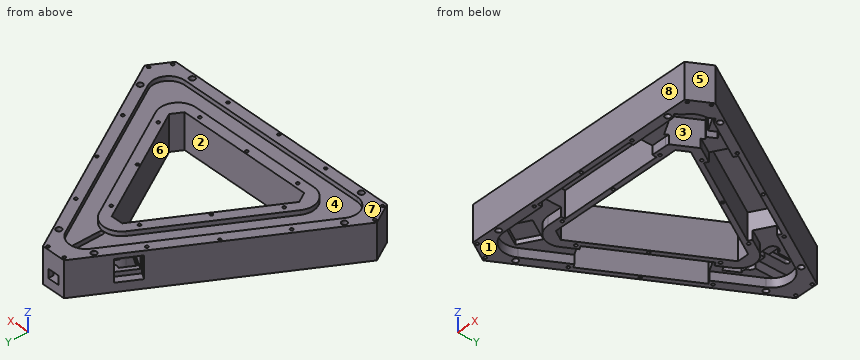
from build123d import *

# Parameters (mm, degrees)
PAD_DEPTH             = 24
POCKET_DEPTH          = 3
SKETCH002_W           = 70
SKETCH002_H           = 18.5
POCKET001_DEPTH       = 18
POLARPATTERN_COUNT    = 3
POCKET002_DEPTH       = 6
CHAMFER_SIZE          = 8
FILLET_R              = 13
FILLET001_R           = 11
CHAMFER001_SIZE       = 16.1
FILLET002_R           = 11
FILLET003_R           = 12
POCKET003_DEPTH       = 6
POCKET004_DEPTH       = 18
POCKET005_DEPTH       = 21.001
SKETCH007_W           = 15.5
SKETCH007_H           = 15
POCKET006_DEPTH       = 5
SKETCH010_W           = 13.6
SKETCH010_H           = 9
POCKET009_DEPTH       = 15.5
POCKET010_DEPTH       = 3
SKETCH012_R           = 1.85
SKETCH012_R_2         = 0.99
POCKET011_DEPTH       = 498.0492855781
POLARPATTERN001_COUNT = 3
POCKET012_DEPTH       = 12
POCKET013_DEPTH       = 3
POCKET014_DEPTH       = 3
FILLET004_R           = 0.6
FILLET005_R           = 2.6


with BuildPart() as part:
    # Sketch → Pad (new body)
    with BuildSketch(Plane.XY):
        Polygon((0, 112.2094915052), (-97.1762701892, -56.1047457526), (97.1762701892, -56.1047457526), align=None)
        Polygon((0, 62.2094915052), (-53.875, -31.1047457526), (53.875, -31.1047457526), align=None, mode=Mode.SUBTRACT)
    extrude(amount=PAD_DEPTH)

    # Sketch001 (on Face8 of Pad) → Pocket (cut)
    with BuildSketch(Plane.XY.offset(24)):
        Polygon((0, 98.2094915052), (-85.0519145362, -49.1047457526), (85.0519145362, -49.1047457526), align=None)
        Polygon((0, 76.2094915052), (-65.999355653, -38.1047457526), (65.999355653, -38.1047457526), align=None, mode=Mode.SUBTRACT)
    extrude(amount=-POCKET_DEPTH, mode=Mode.SUBTRACT)

    # Sketch002 (on Face4 of Pocket) → Pocket001 (cut)
    with BuildSketch(Plane(origin=(0, 0, 0), x_dir=(1, 0, 0), z_dir=(0, 0, -1))):
        with Locations((0, 43.6047457526)):
            Rectangle(SKETCH002_W, SKETCH002_H)
    pocket001 = extrude(amount=-POCKET001_DEPTH, mode=Mode.SUBTRACT)

    # PolarPattern: Pocket001 ×3 about axis
    polarpattern_axis = Axis((0, 0, 0), (0, 0, -1))
    for i in range(1, POLARPATTERN_COUNT):
        add(pocket001.rotate(polarpattern_axis, i * 360 / POLARPATTERN_COUNT), mode=Mode.SUBTRACT)

    # Sketch003 (on Face4 of PolarPattern) → Pocket002 (cut)
    with BuildSketch(Plane(origin=(0, 0, 0), x_dir=(1, 0, 0), z_dir=(0, 0, -1))):
        Polygon((0, -100.2094915052), (86.7839653438, 50.1047457526), (-86.7839653438, 50.1047457526), align=None)
        Polygon((0, -74.2094915052), (64.2673048454, 37.1047457526), (-64.2673048454, 37.1047457526), align=None, mode=Mode.SUBTRACT)
    extrude(amount=-POCKET002_DEPTH, mode=Mode.SUBTRACT)

    # Chamfer
    chamfer_edges = [part.edges().sort_by_distance(p)[0] for p in [
        (-53.875, -31.104746, 12),
        (53.875, -31.104746, 12),
        (0, 62.209492, 12),
    ]]
    chamfer(chamfer_edges, length=CHAMFER_SIZE)

    # Fillet
    fillet_edges = [part.edges().sort_by_distance(p)[0] for p in [
        (0, 100.209492, 3),
        (-86.783965, -50.104746, 3),
        (86.783965, -50.104746, 3),
    ]]
    fillet(fillet_edges, radius=FILLET_R)

    # Fillet001
    fillet001_edges = [part.edges().sort_by_distance(p)[0] for p in [
        (0, 74.209492, 3),
        (64.267305, -37.104746, 3),
        (-64.267305, -37.104746, 3),
    ]]
    fillet(fillet001_edges, radius=FILLET001_R)

    # Chamfer001
    chamfer001_edges = [part.edges().sort_by_distance(p)[0] for p in [
        (97.17627, -56.104746, 12),
        (0, 112.209492, 12),
        (-97.17627, -56.104746, 12),
    ]]
    chamfer(chamfer001_edges, length=CHAMFER001_SIZE)

    # Fillet002
    fillet002_edges = [part.edges().sort_by_distance(p)[0] for p in [
        (0, 98.209492, 22.5),
        (-85.051915, -49.104746, 22.5),
        (85.051915, -49.104746, 22.5),
    ]]
    fillet(fillet002_edges, radius=FILLET002_R)

    # Fillet003
    fillet003_edges = [part.edges().sort_by_distance(p)[0] for p in [
        (65.999356, -38.104746, 22.5),
        (0, 76.209492, 22.5),
        (-65.999356, -38.104746, 22.5),
    ]]
    fillet(fillet003_edges, radius=FILLET003_R)

    # Sketch004 (on Face60 of Fillet003) → Pocket003 (cut)
    with BuildSketch(Plane(origin=(0, 0, 6), x_dir=(1, 0, 0), z_dir=(0, 0, -1))):
        Polygon((-8.75, -71.2664825043), (8.75, -71.2664825043), (8.75, -94.7664825043), (4, -94.7664825043), (4, -98.2664825043), (-4, -98.2664825043), (-4, -94.7664825043), (-8.75, -94.7664825043), align=None)
    extrude(amount=-POCKET003_DEPTH, mode=Mode.SUBTRACT)

    # Sketch005 (on Face29 of Pocket003) → Pocket004 (cut)
    with BuildSketch(Plane(origin=(0, 0, 0), x_dir=(1, 0, 0), z_dir=(0, 0, -1))):
        Polygon((46.1715988394, 38.9547457526), (68.6882593378, 51.9547457526), (79.3382593378, 33.508404652), (56.8215988394, 20.508404652), align=None)
    extrude(amount=-POCKET004_DEPTH, mode=Mode.SUBTRACT)

    # Sketch006 (on Face1 of Pocket004) → Pocket005 (cut, through all)
    with BuildSketch(Plane.XY.offset(21)):
        with BuildLine():
            ThreePointArc((1.5, 85.0404521425), (0, 86.5404521425), (-1.5, 85.0404521425))
            Line((-1.5, 85.0404521425), (-1.5, 66.0404521425))
            ThreePointArc((-1.5, 66.0404521425), (0, 64.5404521425), (1.5, 66.0404521425))
            Line((1.5, 85.0404521425), (1.5, 66.0404521425))
        make_face()
    extrude(amount=-POCKET005_DEPTH, mode=Mode.SUBTRACT)

    # Sketch007 (on Face24 of Pocket005) → Pocket006 (cut)
    with BuildSketch(Plane(origin=(-48.5881350946, 28.0523728763, 0), x_dir=(-0.5, -0.8660254038, 0), z_dir=(-0.8660254038, 0.5, 0))):
        with Locations((-47.3262701892, 13.5)):
            Rectangle(SKETCH007_W, SKETCH007_H)
    extrude(amount=-POCKET006_DEPTH, mode=Mode.SUBTRACT)

    # Sketch010 (on Face79 of Pocket006) → Pocket009 (cut)
    with BuildSketch(Plane(origin=(-44.2580080757, 25.5523728763, 0), x_dir=(-0.5, -0.8660254038, 0), z_dir=(-0.8660254038, 0.5, 0))):
        with Locations((-47.3262701892, 13.5)):
            Rectangle(SKETCH010_W, SKETCH010_H)
    extrude(amount=-POCKET009_DEPTH, mode=Mode.SUBTRACT)

    # Sketch011 (on Face21 of Pocket009) → Pocket010 (cut)
    with BuildSketch(Plane(origin=(0, 0, 6), x_dir=(1, 0, 0), z_dir=(0, 0, -1))):
        Polygon((-21.0413798427, -59.7570681827), (-11.6817654684, -54.3532923042), (-6.658482036, -63.0538744299), (-16.0180964103, -68.4576503084), align=None)
    extrude(amount=-POCKET010_DEPTH, mode=Mode.SUBTRACT)

    # Sketch012 (on Face54 of Pocket010) → Pocket011 (cut, through all)
    with BuildSketch(Plane(origin=(0, 0, 0), x_dir=(1, 0, 0), z_dir=(0, 0, -1))):
        with Locations((-13.5, -82.7032108255)):
            Circle(SKETCH012_R)
        with Locations((13.5, -82.7032108255)):
            Circle(SKETCH012_R)
        with Locations((-6.25, -96.5164825043)):
            Circle(SKETCH012_R_2)
        with Locations((6.25, -96.5164825043)):
            Circle(SKETCH012_R_2)
        with Locations((-27.2463245869, -59.0174730012)):
            Circle(SKETCH012_R_2)
        with Locations((-47.1862074814, -27.2405827309)):
            Circle(SKETCH012_R_2)
        with Locations((-64.7337931796, 5.9127272486)):
            Circle(SKETCH012_R_2)
        with Locations((-10.791841915, -49.5174730012)):
            Circle(SKETCH012_R_2)
        with Locations((-28.3394276132, -16.3641630217)):
            Circle(SKETCH012_R_2)
        with Locations((-48.2793105078, 15.4127272487)):
            Circle(SKETCH012_R_2)
    pocket011 = extrude(amount=-POCKET011_DEPTH, mode=Mode.SUBTRACT)

    # PolarPattern001: Pocket011 ×3 about axis
    polarpattern001_axis = Axis((0, 0, 0), (0, 0, -1))
    for i in range(1, POLARPATTERN001_COUNT):
        add(pocket011.rotate(polarpattern001_axis, i * 360 / POLARPATTERN001_COUNT), mode=Mode.SUBTRACT)

    # Sketch013 (on Face132 of PolarPattern001) → Pocket012 (cut)
    with BuildSketch(Plane(origin=(0, 0, 6), x_dir=(1, 0, 0), z_dir=(0, 0, -1))):
        Polygon((58.553649647, 21.508404652), (63.3167893678, 24.258404652), (66.3167893678, 19.0622522293), (61.553649647, 16.3122522293), align=None)
    extrude(amount=-POCKET012_DEPTH, mode=Mode.SUBTRACT)

    # Sketch014 (on Face127 of Pocket012) → Pocket013 (cut)
    with BuildSketch(Plane(origin=(0, 0, 6), x_dir=(1, 0, 0), z_dir=(0, 0, -1))):
        Polygon((-74.3478338252, 33.3748379063), (-65.8478338252, 48.0972697706), (-52.8574527684, 40.5972697706), (-61.3574527684, 25.8748379063), align=None)
    extrude(amount=-POCKET013_DEPTH, mode=Mode.SUBTRACT)

    # Sketch015 (on Face21 of Pocket013) → Pocket014 (cut)
    with BuildSketch(Plane(origin=(0, 0, 6), x_dir=(1, 0, 0), z_dir=(0, 0, -1))):
        with BuildLine():
            ThreePointArc((-8.75, -64.2614128894), (-12.2525348074, -67.7639476968), (-8.75, -71.2664825043))
            Line((-8.75, -71.2664825043), (8.73, -71.2664825043))
            ThreePointArc((8.73, -71.2664825043), (12.2325348074, -67.7639476968), (8.73, -64.2614128894))
            Line((-8.75, -64.2614128894), (8.73, -64.2614128894))
        make_face()
    extrude(amount=-POCKET014_DEPTH, mode=Mode.SUBTRACT)

    # Fillet004
    fillet004_edges = [part.edges().sort_by_distance(p)[0] for p in [
        (-8.75, 64.261413, 7.5),
    ]]
    fillet(fillet004_edges, radius=FILLET004_R)

    # Fillet005
    fillet005_edges = [part.edges().sort_by_distance(p)[0] for p in [
        (-11.783284, 66.01268, 7.5),
    ]]
    fillet(fillet005_edges, radius=FILLET005_R)


solid = part.part
Input: part model. Units: mm. Frame: model coordinates. Face numbers are marked on the shaded views. A direction names the side the tool comes from. Coordinates: 2 decimals unless noted, no trailing zeros. Write each loop counter-clockwise with the first axis right and the second up, starting at its lowest first coordinate (ties: lowest second). Pieces come first, ordered by that corner, then holes. Notation, with made-up numbers: M 10.5,-19.5 L 36.5,-19.5 A29 ccw 36.5,11.5 Z; hole C 22,-2.75 d11. An arc over 180 degrees is marked long. Answer as a JSON object with one key per item and string values. Group by question number.
(1) Set-up query: the marked faces 1, 2, 3, 4 and 5. Return all of +Z, -Z, +X, -X, +Y, -Y with unobstructed straight access to the full face (end or side cutting, diameter ignored); none if empty.
(2) Section A-A on x = -41.5. Output: boundary loops of the cut face in (y, z).
(3) Contact query for flat-ended pins moving along their axis: P1, Ø8, axis at y = 36.5, z = 6, coming from the +X side; P2, Ø12, axis at y = -7.5, z = 8.5, coming from the +X side; P3, Ø13, axis at y = 80, z = 13.5, coming from the -X side. Output: stop coordinate, or through.
(4) Ray query, line 1 along X through (y, z) = (-25, 22.25); line 2 along Y through (x, z) = (20.5, 22); line 3 along X through (y, z) = (22.5, 2.25). Return the intervals inside material, ascending. Write a range as [from, to].
(5) Section B-B on z = 3. Give the number of separate pieces and of enclosed holes in the cut face, plus the area to 3 significant figures.
(6) Mould query, pull axis Y, two halves, no side actions, for the marked faces 6, 7 and 8. Classes: pulls with the +Y half, pulls with the -Y half, needs draft (parallel to the pull), parting line crosses it, or undercut.
Result set:
{
 "1": {"face 1": "-Z, +X, -X, +Y, -Y", "face 2": "+Z, -Z", "face 3": "-Z", "face 4": "+Z", "face 5": "+Z, -Z, +X, -Y"},
 "2": {"outline": "M -56.1,0 L -50.1,0 L -50.1,6 L -37.1,6 L -37.1,0 L -31.1,0 L -31.1,24 L -38.1,24 L -38.1,21 L -49.1,21 L -49.1,24 L -56.1,24 Z; M -9.67,0 L -3.17,0 L -3.17,18 L 33.83,18 L 33.83,0 L 40.33,0 L 40.33,24 L 26.33,24 L 26.33,21 L 4.33,21 L 4.33,24 L -9.67,24 Z"},
 "3": {"P1": "stops at x = 46.02", "P2": "stops at x = 72.58", "P3": "stops at x = -21.05"},
 "4": {"line 1": "x = [-79.22, -71.14], [-57.16, -49.4], [49.4, 57.16], [71.14, 79.22]", "line 2": "y = [-56.1, -49.1], [-38.1, -31.1], [26.7, 40.7], [62.7, 76.7]", "line 3": "x = [-51.79, -48.04], [-26.68, -22.93], [22.93, 26.68], [48.04, 51.79]"},
 "5": {"separate pieces": "2", "enclosed holes": "32", "area": "3,930 mm2"},
 "6": {"face 6": "undercut", "face 7": "needs draft", "face 8": "pulls with the -Y half"}
}
